```python
from build123d import *

# Parameters (mm, degrees)
BOSS_EXTRUDE2_DEPTH = 10


with BuildPart() as part:
    # Sketch1 → Boss-Extrude2 (new body)
    with BuildSketch(Plane.XY):
        Polygon((13.439595942, -2.441270434), (8.753924566, 10.322427453), (-4.642597738, 12.646365952), (-13.353448667, 2.206606563), (-8.667777292, -10.557091324), (4.728745013, -12.881029823), align=None)
        with BuildLine():
            Line((-1.865402523, -2.496453358), (-1.379890953, 2.580384094))
            ThreePointArc((-1.379890953, 2.580384094), (3.079221525, -0.407686894), (-1.865402523, -2.496453358))
        make_face(mode=Mode.SUBTRACT)
    extrude(amount=BOSS_EXTRUDE2_DEPTH)


solid = part.part
```
Source: CAD feature listing. Evaluate the final solid. Frame: model axes, mm. A direction names the side the tool comes from. Coordinates: 2 decimals unless noted, no trailing zeros. Write each loop counter-clockwise with the first axis right and the second up, starting at its lowest first coordinate (ties: lowest second). Pieces come first, ordered by that corner, then holes. Notation, with made-up numbers: (7, -6.5) - (52, -6.5) arc R17 cw to (52, 13.5) - close; hole circle Ø3 at (45.5, 12.5). An arc over 180 degrees is marked (long way). Answer as a JSON object with one key per item and string values.
Q1. Section query C-C, the plane y = -0.5. Output: boundary loops of the cut face in (x, z).
Ans:
{"outline": "(-12.36, 0) - (-1.67, 0) - (-1.67, 10) - (-12.36, 10) - close; (3.07, 0) - (12.73, 0) - (12.73, 10) - (3.07, 10) - close"}
Q2. Section query A-A, the plane z = 7.25. Output: boundary loops of the cut face in (x, y).
Ans:
{"outline": "(-13.35, 2.21) - (-8.67, -10.56) - (4.73, -12.88) - (13.44, -2.44) - (8.75, 10.32) - (-4.64, 12.65) - close; hole (-1.87, -2.5) arc R3.05 ccw (long way) to (-1.38, 2.58) - close"}
Q3. Draft query along X for faces 1 (the flat face through (-3, 0, 10)), 2 (the cylindrical face through (3.087, -0.316, 4.93)), 3 (the flat face through (11.13, 3.85, 4.93)), 4 (the flat face through (-8.937, 7.5, 4.93)). Return one class per face: released by +X, released by -X, zero draft, split by the parting line, or undercut.
Ans:
{"face 1": "zero draft", "face 2": "undercut", "face 3": "released by +X", "face 4": "released by -X"}
Q4. Material intervals for line 1 (Y direction, x = 2.5, z = 1); line 2 (X direction, y = 0.25, z = 4.25); line 3 (X direction, y = -1, z = 0.5), sorted ascending. Write a range as [from, to].
Ans:
{"line 1": "y = [-12.49, -1.92], [1.69, 11.41]", "line 2": "x = [-12.64, -1.6], [3.07, 12.45]", "line 3": "x = [-12.18, -1.72], [2.96, 12.91]"}
Q5. Section query D-D, the plane y = -5.75. Output: boundary loops of the cut face in (x, z), plus the area to 3 significant figures.
Ans:
{"outline": "(-10.43, 0) - (10.68, 0) - (10.68, 10) - (-10.43, 10) - close", "area": "211 mm2"}
Q6. Section query B-B, the plane x = 2.5. Output: boundary loops of the cut face in (y, z), plus the area to 3 significant figures.
Ans:
{"outline": "(-12.49, 0) - (-1.92, 0) - (-1.92, 10) - (-12.49, 10) - close; (1.69, 0) - (11.41, 0) - (11.41, 10) - (1.69, 10) - close", "area": "203 mm2"}
Q7. First-contact query: pin 1 Ø6 at (y, z) = (2.5, 6.5) entering from -X; pin 2 Ø3 at (y, z) = (-7, 3.5) entering from -X. Flat tips, straight axial feed; report the tip coordinate or a pass-through.
Ans:
{"pin 1": "stops at x = -13.35", "pin 2": "stops at x = -10.52"}
Q8. Set-up query: faces 5 (the flat face through (-1.626, 0.006, 4.93)), 6 (the flat face through (2.15, 11.47, 4.93)). Return all of +Z, -Z, +X, -X, +Y, -Y with unobstructed straight access to the full face (end or side cutting, diameter ignored); none if empty.
Ans:
{"face 5": "+Z, -Z", "face 6": "+Z, -Z, +X, +Y"}
